Autodesk Inventor part; units mm, degrees
ref_plane "YZ Plane" through (0, 0, 0) normal (1, 0, 0) x (0, 1, 0)
ref_plane "XZ Plane" through (0, 0, 0) normal (0, 1, 0) x (-1, 0, 0)
ref_plane "XY Plane" through (0, 0, 0) normal (0, 0, 1) x (1, 0, 0)
sketch "Sketch1" plane through (0, 0, 0) normal (0, 0, 1) x (1, 0, 0)
  line L0 (-20.1958, -14.566) -> (13.8042, -14.566)
  line L1 (13.8042, -14.566) -> (13.8042, 14.434)
  line L2 (13.8042, 14.434) -> (-20.1958, 14.434)
  line L3 (-20.1958, 14.434) -> (-20.1958, -14.566)
  circle A0 centre (11.3042, 9.934) radius 1.5
  circle A1 centre (11.3042, -10.066) radius 1.5
  circle A2 centre (-17.3958, 9.934) radius 1.5
  circle A3 centre (-17.3958, -10.066) radius 1.5
  point P0 (0, 0)
  dimension "d1" = 34
  dimension "d2" = 3
  dimension "d3" = 3
  dimension "d4" = 20
  dimension "d5" = 3
  dimension "d6" = 3
  dimension "d8" = 28.7
  dimension "d9" = 2.5
  dimension "d10" = 20
  dimension "d11" = 29
  dimension "d12" = 4.5
extrude "Extrusion1" add sketch "Sketch1" along normal blind 5
thread "Thread1"
thread "Thread2"
thread "Thread3"
thread "Thread4"
sketch "Sketch3" plane through (0, 0, 5) normal (0, 0, 1) x (1, 0, 0)
  line L0 (-9.0293, 4.1042) -> (2.8565, 4.1042) construction
  line L1 (2.8565, 4.1042) -> (2.8565, -3.7102) construction
  line L2 (2.8565, -3.7102) -> (-9.0293, -3.7102) construction
  line L3 (-9.0293, -3.7102) -> (-9.0293, 4.1042) construction
  point P0 (0, 0)
  dimension "d3" = 3
properties material "ABS Plastic"
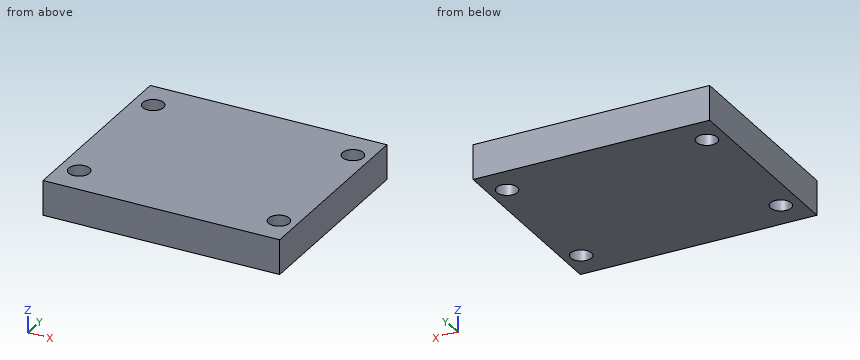
The listing builds one solid part. Answer for the finished solid, in the listing's coordinates (mm). Round coordinates to 2 decimals unless told otherwise and drop trailing zeros. Write each loop counter-clockwise with the first axis right and the second up, starting at its lowest first coordinate (ties: lowest second). Pieces come first, ordered by that corner, then holes. Notation, with made-up numbers: (50.5, 41.25) -> (104.5, 41.25) arc R20 ccw to (104.5, 46.25) -> close; hole circle Ø1 at (-20, 10.5). An arc over 180 degrees is marked (long way). Use CSV: the item, a comma, the result in double quotes. Start each with the question number.
(1) Section B-B on z = 1.4 is taken. Give the vertices of the cut face in (x, y), then the cut area to 3 significant figures.
(2) Section A-A on y = 9 is taken. Give the vertices of the cut face in (x, z).
(3) Consider L1, parallel to Y at x = -17.5, z = 3; L2, parallel to Y at x = 10, z = 2.45; L3, parallel to X at y = -8.75, z = 0.6. Determine where each line is inside the solid, lowest interval first. Write a range as from..to.
A:
1,outline,"(-20.2, -14.57) -> (13.8, -14.57) -> (13.8, 14.43) -> (-20.2, 14.43) -> close; hole circle Ø3 at (-17.4, -10.07); hole circle Ø3 at (-17.4, 9.93); hole circle Ø3 at (11.3, -10.07); hole circle Ø3 at (11.3, 9.93)"
1,area,"958 mm²"
2,outline,"(-20.2, 0) -> (-18.57, 0) -> (-18.57, 5) -> (-20.2, 5) -> close; (-16.22, 0) -> (10.13, 0) -> (10.13, 5) -> (-16.22, 5) -> close; (12.48, 0) -> (13.8, 0) -> (13.8, 5) -> (12.48, 5) -> close"
3,L1,"y = -14.57..-11.56, -8.57..8.44, 11.43..14.43"
3,L2,"y = -14.57..-10.81, -9.33..9.19, 10.67..14.43"
3,L3,"x = -20.2..-18.12, -16.68..10.58, 12.02..13.8"
